Design review of the part shown in the three views and the two pictorial views. Dimensions are in mm from the part's minimum x, y and z. A direction names the side the tool comes from. Give positions to 0.01 mm unless a question says otherwise; leave off trailing zeros. Loops run counter-clockwise (first coordinate to the right, second up) from the corner with the lowest first, then second, coordinate; pieces in that order, holes last. Notation, with made-up numbers: (-12, -21) -> (12, -21) arc R20 cw to (12, -12) -> close; hole circle Ø2 at (27, -26.75). An arc over 180 degrees is marked (long way). Answer as CSV lines item,"result".
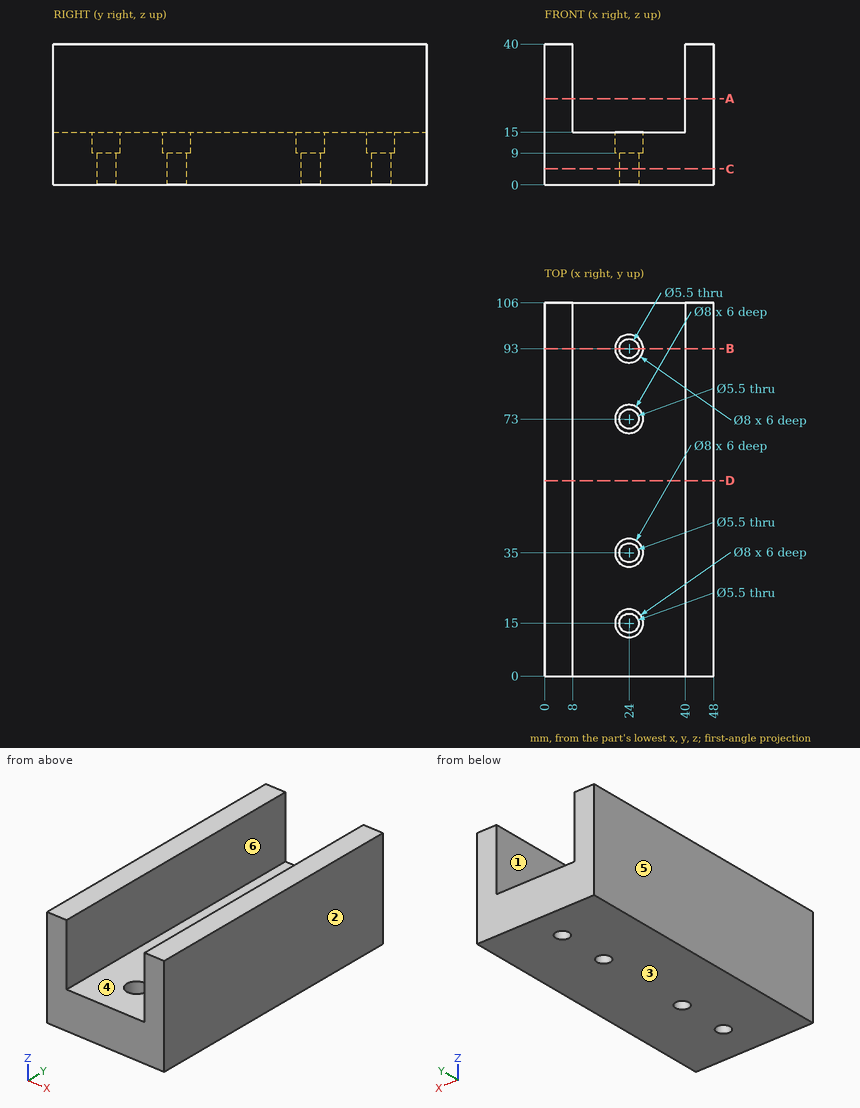
Q1. To check wall thickness, follow probe 1 along Y at (x, z) = (24, 4.5); probe 2 along Y at (x, z) = (24, 12); probe 3 along X at (y, z) = (15.5, 19). State the ranges of each line that lie inside material, in increasing order. Write a range as from..to.
Filled sheet:
probe 1,"y = 0..12.25, 17.75..32.25, 37.75..70.25, 75.75..90.25, 95.75..106"
probe 2,"y = 0..11, 19..31, 39..69, 77..89, 97..106"
probe 3,"x = 0..8, 40..48"
Q2. We need section C-C, the plane z = 4.5. State the section outline as (x, y) points.
Filled sheet:
outline,"(0, 0) -> (48, 0) -> (48, 106) -> (0, 106) -> close; hole circle Ø5.5 at (24, 15); hole circle Ø5.5 at (24, 35); hole circle Ø5.5 at (24, 73); hole circle Ø5.5 at (24, 93)"
Q3. We need section A-A, the plane z = 24.5. State the section outline as (x, y) points, and give its area (3 significant figures).
Filled sheet:
outline,"(0, 0) -> (8, 0) -> (8, 106) -> (0, 106) -> close; (40, 0) -> (48, 0) -> (48, 106) -> (40, 106) -> close"
area,"1,700 mm^2"
Q4. The part is to be moulded in two halves that separate along X. For the marked faces 1, 2, 3 and 4, say which applies: pulls with the +X half, pulls with the -X half, needs draft (parallel to the pull), parting line crosses it, or undercut.
Filled sheet:
face 1,"undercut"
face 2,"pulls with the +X half"
face 3,"needs draft"
face 4,"undercut"
Q5. We need section B-B, the plane y = 93. State the section outline as (x, z) points.
Filled sheet:
outline,"(0, 0) -> (21.25, 0) -> (21.25, 9) -> (20, 9) -> (20, 15) -> (8, 15) -> (8, 40) -> (0, 40) -> close; (26.75, 0) -> (48, 0) -> (48, 40) -> (40, 40) -> (40, 15) -> (28, 15) -> (28, 9) -> (26.75, 9) -> close"
Q6. We need section D-D, the plane y = 55.5. State the section outline as (x, z) points, and give its area (3 significant figures).
Filled sheet:
outline,"(0, 0) -> (48, 0) -> (48, 40) -> (40, 40) -> (40, 15) -> (8, 15) -> (8, 40) -> (0, 40) -> close"
area,"1,120 mm^2"
Q7. For the marked faces 5 and 6, list the 3-axis set-ups (+Z, -Z, +X, -X, +Y, -Y) from which the entire face can be reached by the end or side of a thin tool; tool diameter is ignored.
Filled sheet:
face 5,"+Z, -Z, -X, +Y, -Y"
face 6,"+Z, +Y, -Y"
Q8. Clearance check with flat-ended pins moving along their axes: pin 1 Ø9 at (x, y) = (24, 33) entering from +Z; pin 2 Ø6.5 at (x, y) = (24, 15) entering from +Z. State where each tip first meets the part, or that it passes through.
Filled sheet:
pin 1,"stops at z = 15"
pin 2,"stops at z = 9"
